from build123d import *

# Parameters (mm, degrees)
SKETCH1_W           = 103
SKETCH1_H           = 69
BOSS_EXTRUDE1_DEPTH = 3
SKETCH2_W           = 81
SKETCH2_H           = 47
CUT_EXTRUDE1_DEPTH  = 3
CUT_EXTRUDE2_DEPTH  = 2
FILLET2_R           = 2.5
FILLET3_R           = 2.5
CHAMFER1_SIZE       = 0.5
CUT_EXTRUDE3_DEPTH  = 2
SKETCH5_W           = 10
SKETCH5_H           = 2
BOSS_EXTRUDE2_DEPTH = 7.5
SKETCH6_W           = 10
SKETCH6_H           = 5.85
BOSS_EXTRUDE3_DEPTH = 7.5
BOSS_EXTRUDE4_DEPTH = 10
BOSS_EXTRUDE5_DEPTH = 10
SKETCH9_W           = 5.55
SKETCH9_H           = 2.55
CUT_EXTRUDE4_DEPTH  = 6.5
SKETCH10_R          = 1.875
CUT_EXTRUDE5_DEPTH  = 1.65


with BuildPart() as part:
    # Sketch1 → Boss-Extrude1 (new body)
    with BuildSketch(Plane.XY):
        with Locations((62.328366078, 28.443882797)):
            Rectangle(SKETCH1_W, SKETCH1_H)
    extrude(amount=BOSS_EXTRUDE1_DEPTH)

    # Sketch2 → Cut-Extrude1 (cut)
    with BuildSketch(Plane.XY.offset(3)):
        with Locations((62.328366078, 28.443882797)):
            Rectangle(SKETCH2_W, SKETCH2_H)
    extrude(amount=-CUT_EXTRUDE1_DEPTH, mode=Mode.SUBTRACT)

    # Sketch3 → Cut-Extrude2 (cut)
    with BuildSketch(Plane.XY.offset(3)):
        Polygon((13.078366078, 55.093882797), (106.378366078, 55.093882797), (106.378366078, 1.793882797), (13.078366078, 1.793882797), (13.078366078, 20.043882797), (11.578366078, 20.043882797), (11.578366078, 36.043882797), (13.078366078, 36.043882797), align=None)
    extrude(amount=-CUT_EXTRUDE2_DEPTH, mode=Mode.SUBTRACT)

    # Fillet2
    fillet2_edges = [part.edges().sort_by_distance(p)[0] for p in [
        (113.828366078, -6.056117203, 1.5),
        (10.828366078, -6.056117203, 1.5),
        (10.828366078, 62.943882797, 1.5),
        (113.828366078, 62.943882797, 1.5),
    ]]
    fillet(fillet2_edges, radius=FILLET2_R)

    # Fillet3
    fillet3_edges = [part.edges().sort_by_distance(p)[0] for p in [
        (21.828366078, 4.943882797, 0.5),
        (21.828366078, 51.943882797, 0.5),
        (102.828366078, 51.943882797, 0.5),
        (102.828366078, 4.943882797, 0.5),
    ]]
    fillet(fillet3_edges, radius=FILLET3_R)

    # Chamfer1
    chamfer1_edges = [part.edges().sort_by_distance(p)[0] for p in [
        (22.560599125, 51.21164975, 0),
        (22.560599125, 5.676115844, 0),
        (102.096133031, 5.676115844, 0),
        (102.096133031, 51.21164975, 0),
        (21.828366078, 28.443882797, 0),
        (62.328366078, 51.943882797, 0),
        (62.328366078, 4.943882797, 0),
        (102.828366078, 28.443882797, 0),
    ]]
    chamfer(chamfer1_edges, length=CHAMFER1_SIZE)

    # Sketch4 → Cut-Extrude3 (cut)
    with BuildSketch(Plane.XY.offset(3)):
        Polygon((16.728366078, 55.093882797), (16.728366078, 56.943882797), (12.728366078, 56.943882797), (12.728366078, 51.943882797), (13.078366078, 51.943882797), (13.078366078, 55.093882797), align=None)
        Polygon((103.728366078, 55.093882797), (103.728366078, 57.443882797), (108.728366078, 57.443882797), (108.728366078, 52.443882797), (106.378366078, 52.443882797), (106.378366078, 55.093882797), align=None)
        Polygon((16.728366078, 1.793882797), (16.728366078, -0.056117203), (12.728366078, -0.056117203), (12.728366078, 3.943882797), (13.078366078, 3.943882797), (13.078366078, 1.793882797), align=None)
        Polygon((103.728366078, 1.793882797), (103.728366078, -0.556117203), (108.728366078, -0.556117203), (108.728366078, 4.443882797), (106.378366078, 4.443882797), (106.378366078, 1.793882797), align=None)
    extrude(amount=-CUT_EXTRUDE3_DEPTH, mode=Mode.SUBTRACT)

    # Sketch5 → Boss-Extrude2 (add)
    with BuildSketch(Plane.XY.offset(3)):
        with Locations((84.228366078, 59.693882797)):
            Rectangle(SKETCH5_W, SKETCH5_H)
        with Locations((40.228366078, 59.693882797)):
            Rectangle(SKETCH5_W, SKETCH5_H)
    extrude(amount=BOSS_EXTRUDE2_DEPTH)

    # Sketch6 → Boss-Extrude3 (add)
    with BuildSketch(Plane.XY.offset(3)):
        with Locations((86.328366078, -1.131117203)):
            Rectangle(SKETCH6_W, SKETCH6_H)
        with Locations((38.328366078, -1.131117203)):
            Rectangle(SKETCH6_W, SKETCH6_H)
    extrude(amount=BOSS_EXTRUDE3_DEPTH)

    # Sketch7 → Boss-Extrude4 (add)
    with BuildSketch(Plane.ZY.offset(-35.228366078)):
        Polygon((7.5, 60.693882797), (7.5, 61.943882797), (10.5, 60.693882797), align=None)
        Polygon((3, 57.693882797), (6.75, 58.693882797), (3, 58.693882797), align=None)
    extrude(amount=-BOSS_EXTRUDE4_DEPTH)

    # Sketch8 → Boss-Extrude5 (add)
    with BuildSketch(Plane.ZY.offset(-79.228366078)):
        Polygon((7.5, 60.693882797), (7.5, 61.943882797), (10.5, 60.693882797), align=None)
        Polygon((6.75, 58.693882797), (3, 58.693882797), (3, 57.693882797), align=None)
    extrude(amount=-BOSS_EXTRUDE5_DEPTH)

    # Sketch9 → Cut-Extrude4 (cut)
    with BuildSketch(Plane.XY.offset(10.5)):
        with Locations((86.328366078, -1.131117203)):
            Rectangle(SKETCH9_W, SKETCH9_H)
        with Locations((38.328366078, -1.131117203)):
            Rectangle(SKETCH9_W, SKETCH9_H)
    extrude(amount=-CUT_EXTRUDE4_DEPTH, mode=Mode.SUBTRACT)

    # Sketch10 → Cut-Extrude5 (cut)
    with BuildSketch(Plane.XZ.offset(4.056117203)):
        with Locations(Location((38.328366078, 7.2, 0), (0, 0, 270))):
            Circle(SKETCH10_R)
        with Locations(Location((86.328366078, 7.2, 0), (0, 0, 270))):
            Circle(SKETCH10_R)
    extrude(amount=-CUT_EXTRUDE5_DEPTH, mode=Mode.SUBTRACT)


solid = part.part
Input: part model. Units: mm. Frame: model coordinates. A direction names the side the tool comes from. Round coordinates to 2 decimals unless told otherwise and drop trailing zeros. Write each loop counter-clockwise with the first axis right and the second up, starting at its lowest first coordinate (ties: lowest second). Pieces come first, ordered by that corner, then holes.
1) Ray query, L1, parallel to X at y = -3.05, z = 7.2; L2, parallel to X at y = 60.5, z = 10; L3, parallel to Y at x = 78, z = 1.75. Return the intervals inside material, ascending.
2) Cut plane A-A (y = 47). Return the cut outline in (x, z), then the cut area to 4 significant figures.
3) Cut plane B-B (x = 97.5). Return the cut outline in (y, z), then the cut area to 4 significant figures.
4) Draft query along Y for faces 6 (the flat face through (38, -1, 4)), 7 (the flat face through (38, -4.056, 5)), 8 (the flat face through (113.828, 28, 1)). Return one class per face: pulls with the +Y half, pulls with the -Y half, needs draft (parallel to the pull), parting line crosses it, or undercut.
5) Contact query for flat-ended pins moving along their axis: P1, Ø3, axis at x = 39.5, z = 7, coming from the -Y side; P2, Ø2, axis at y = -1, z = 6, coming from the +X side; P3, Ø3, axis at y = 0, z = 7, coming from the -X side; P4, Ø12, axis at x = 41.5, y = 16, coming from the +Z side. Output: stop coordinate, or through.
6) Reachability of faces 1 (the flat face through (86, -4.056, 5)), 2 (the flat face through (86, -1, 4)), 3 (the flat face through (91.328, -1, 7)), 4 (the flat face through (35.228, 60, 7)), 5 (the flat face through (40.158, 58.187, 4.849)) from +Z, -Z, +X, -X, +Y, -Y: full face, straight path, thin tool, end or side. Return the list, or none.
Geometry says:
1. L1: x = 33.33 to 36.45, 40.2 to 43.33, 81.33 to 84.45, 88.2 to 91.33
1. L2: x = 35.23 to 45.23, 79.23 to 89.23
1. L3: y = -6.06 to 1.79, 55.09 to 62.94
2. outline: (10.83, 0) - (21.33, 0) - (21.83, 0.5) - (21.83, 1) - (13.08, 1) - (13.08, 3) - (10.83, 3) - close; (102.83, 0.5) - (103.33, 0) - (113.83, 0) - (113.83, 3) - (106.38, 3) - (106.38, 1) - (102.83, 1) - close
2. area: 41.15 mm2
3. outline: (-6.06, 0) - (4.44, 0) - (4.94, 0.5) - (4.94, 1) - (1.79, 1) - (1.79, 3) - (-6.06, 3) - close; (51.94, 0.5) - (52.44, 0) - (62.94, 0) - (62.94, 3) - (55.09, 3) - (55.09, 1) - (51.94, 1) - close
3. area: 53.15 mm2
4. face 6: undercut
4. face 7: pulls with the -Y half
4. face 8: needs draft
5. P1: stops at y = -4.06
5. P2: stops at x = 91.33
5. P3: stops at x = 33.33
5. P4: passes through
6. face 1: +Z, +X, -X, -Y
6. face 2: +Z
6. face 3: +Z, +X, +Y, -Y
6. face 4: +Z, -X, +Y
6. face 5: +Z, +X, -X
